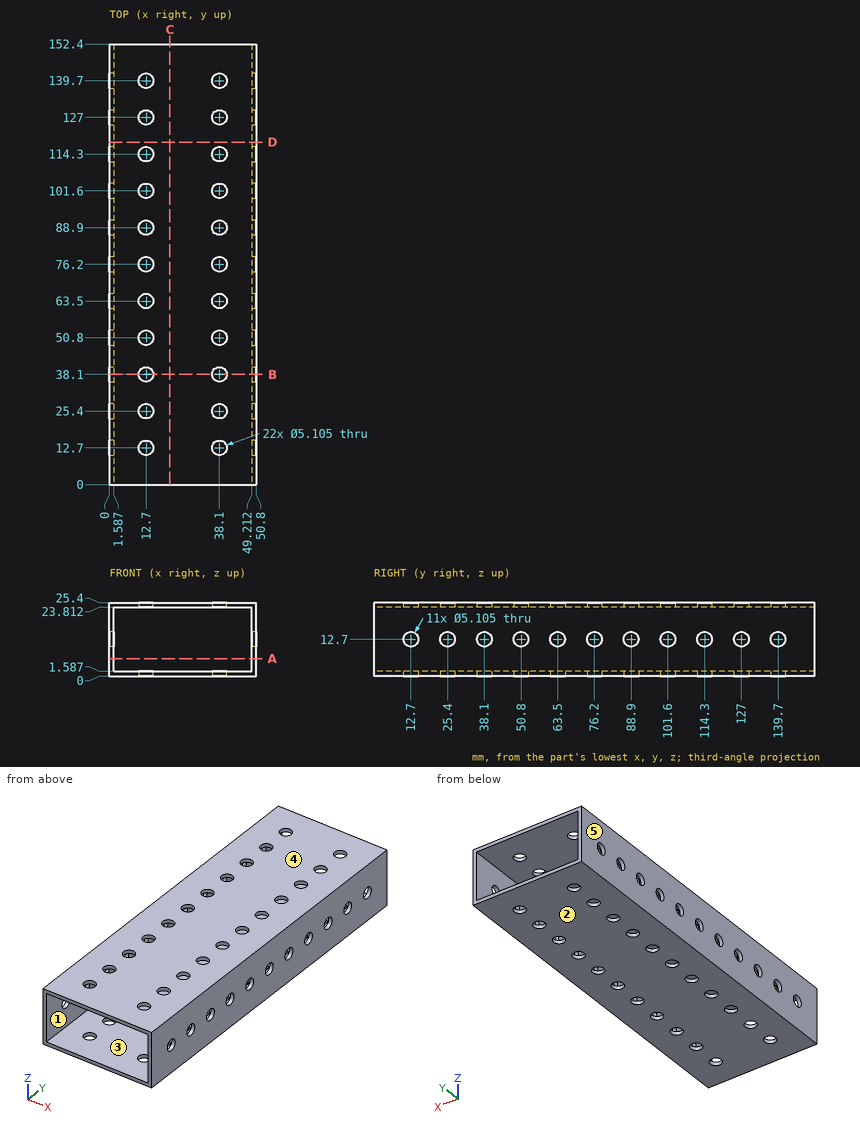
The drawing under review shows one solid part. Ordinate dimensions are in mm from its lowest x, y, z. A direction names the side the tool comes from. Round coordinates to 2 decimals unless told otherwise and drop trailing zeros. Write each loop counter-clockwise with the first axis right and the second up, starting at its lowest first coordinate (ties: lowest second). Pieces come first, ordered by that corner, then holes.
(1) We need section A-A on z = 6. Give the boundary of the cut face in (x, y).
(2) Mouldability with a two-part tool opening along Z and no side actions: class the marked faces 3, 4 and 5 as +Z half, -Z half, draft (parallel to the pull), parting line (faces both ways), or undercut.
(3) We need section D-D on y = 118.5. Give the boundary of the cut face in (x, z).
(4) Machinability: for the marked faces 1 and 2, which of the approach directions +Z, -Z, +X, -X, +Y, -Y give a long, thin tool a straight path to every point of the face, cutting with its end or side? Answer none if there is none.
(5) We need section B-B on y = 38.1. Give the number of separate pieces and of enclosed holes in the cut face, and give its area (3 significant figures).
(6) We need section C-C on x = 21. Give the boundary of the cut face in (y, z).
(7) Wall thickness on L1, parallel to X at y = 63.5, z = 0.35; L2, parallel to X at y = 81.5, z = 23; L3, parallel to Z at x = 20.5, y = 16: over which ranges is each line inside the solid? List them lowest first.
Findings below:
1. outline: (0, 0) - (1.59, 0) - (1.59, 152.4) - (0, 152.4) - close; (49.21, 0) - (50.8, 0) - (50.8, 152.4) - (49.21, 152.4) - close
2. face 3: undercut
2. face 4: +Z half
2. face 5: draft
3. outline: (0, 0) - (50.8, 0) - (50.8, 25.4) - (0, 25.4) - close; hole (1.59, 1.59) - (49.21, 1.59) - (49.21, 23.81) - (1.59, 23.81) - close
4. face 1: +Y, -Y
4. face 2: -Z, +X, -X, +Y, -Y
5. separate pieces: 6
5. enclosed holes: 0
5. area: 183 mm2
6. outline: (0, 0) - (152.4, 0) - (152.4, 1.59) - (0, 1.59) - close; (0, 23.81) - (152.4, 23.81) - (152.4, 25.4) - (0, 25.4) - close
7. L1: x = 0 to 10.15, 15.25 to 35.55, 40.65 to 50.8
7. L2: x = 0 to 1.59, 49.21 to 50.8
7. L3: z = 0 to 1.59, 23.81 to 25.4
